Can you work these out from the drawing? Everything is in mm from the part's minimum corner. A direction names the side the tool comes from. Coordinates: 2 decimals unless noted, no trailing zeros. Order: outer loops, then holes, each group sorted by start corner. A loop starts at its lowest first (then second) coordinate and runs counter-clockwise, first axis right, second up. Notation, with made-up numbers: (-37, 81) - (11, 81) arc R21 ccw to (11, 115) - close; hole circle Ø1 at (60.5, 32.5). An arc over 180 degrees is marked (long way). Answer as CSV lines item,"result". Start each with the question number.
Item 1: I need wall thicknesses on line 1 (Y direction, x = 9.5, z = 3.75) (1 decimal); line 2 (X direction, y = 8, z = 3.7); line 3 (Z direction, x = 41, y = 26). Which ranges of each line are inside material? Lowest first, please.
Item 2: We'd pull the mould along Y, two halves only. Please class the marked faces 3 and 4: pulls with the +Y half, pulls with the -Y half, needs draft (parallel to the pull), parting line crosses it, or undercut.
Item 3: Imagine slicing it at B-B on x = 10. List the corners of the cut face in (y, z) for me (1 decimal), and give its area (3 significant figures).
Item 4: On a 3-axis mill with a long thin cutter (end or side, diameter ignored), from which of +Z, -Z, +X, -X, +Y, -Y can I reach the whole of each face in a straight line? I mean the marked faces 1 and 2. Say none if no direction works.
Item 5: I'm going to push flat-ended pins straight in: pin 1 (1.6 mm diameter, centred on x = 13, z = 1.5, fed in from +Y); pin 2 (0.6 mm diameter, centred on y = 30, z = 1, fed in from -X); pin 3 (1.5 mm diameter, centred on x = 35.5, z = 1, fed in from -Y). Where does each tip first touch, or does it pass through?
Item 6: Imagine slicing it at C-C on z = 3.45. List the corners of the cut face in (x, y) for me (1 decimal).
Item 7: Imagine slicing it at A-A on y = 6.5. List the corners of the cut face in (x, z) for me.
Item 8: Imagine slicing it at D-D on x = 19. List the corners of the cut face in (y, z) for me.
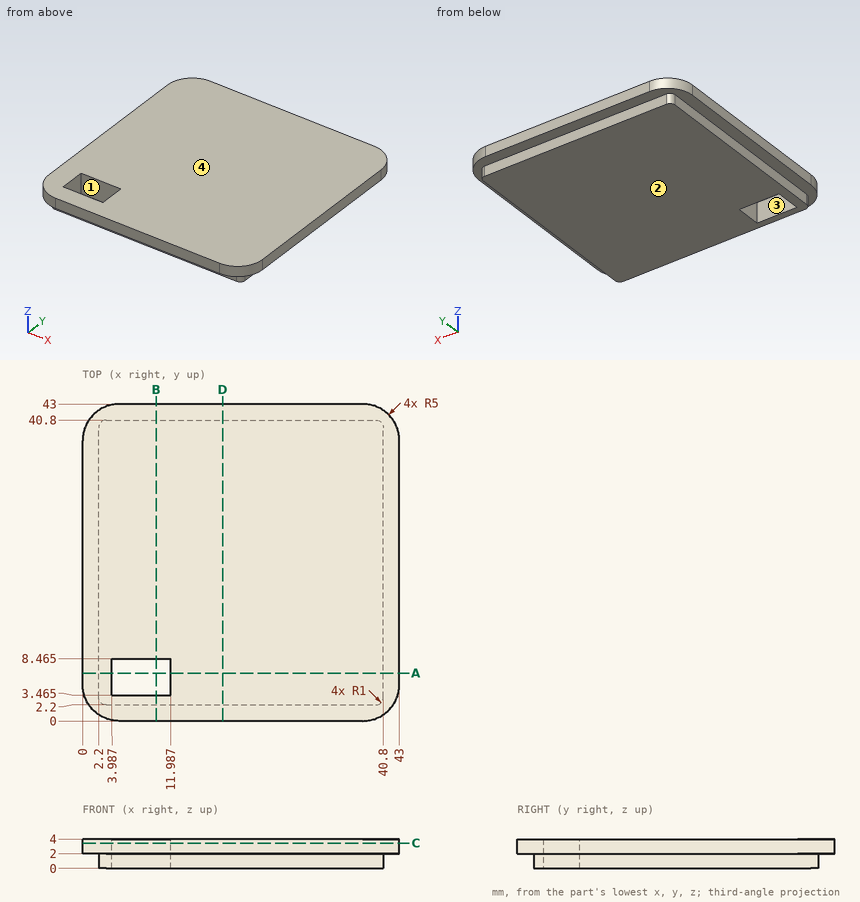
Responses:
1,line 1,"y = 0 to 3.5, 8.5 to 43"
1,line 2,"x = 0 to 3.99, 11.99 to 43"
1,line 3,"z = 2 to 4"
2,face 3,"undercut"
2,face 4,"needs draft"
3,outline,"(0, 2) - (2.2, 2) - (2.2, 0) - (3.5, 0) - (3.5, 4) - (0, 4) - close; (8.5, 0) - (40.8, 0) - (40.8, 2) - (43, 2) - (43, 4) - (8.5, 4) - close"
3,area,"143 mm^2"
4,face 1,"+Z, -Z"
4,face 2,"-Z, +X, -X, +Y, -Y"
5,pin 1,"stops at y = 43"
5,pin 2,"stops at x = 2.2"
5,pin 3,"stops at y = 2.2"
6,outline,"(0, 5) arc R5 ccw to (5, 0) - (38, 0) arc R5 ccw to (43, 5) - (43, 38) arc R5 ccw to (38, 43) - (5, 43) arc R5 ccw to (0, 38) - close; hole (4, 3.5) - (12, 3.5) - (12, 8.5) - (4, 8.5) - close"
7,outline,"(0, 2) - (2.2, 2) - (2.2, 0) - (3.99, 0) - (3.99, 4) - (0, 4) - close; (11.99, 0) - (40.8, 0) - (40.8, 2) - (43, 2) - (43, 4) - (11.99, 4) - close"
8,outline,"(0, 2) - (2.2, 2) - (2.2, 0) - (40.8, 0) - (40.8, 2) - (43, 2) - (43, 4) - (0, 4) - close"
